Autodesk Inventor part; units mm, degrees
ref_plane "YZ Plane" through (0, 0, 0) normal (1, 0, 0) x (0, 1, 0)
ref_plane "XZ Plane" through (0, 0, 0) normal (0, 1, 0) x (-1, 0, 0)
ref_plane "XY Plane" through (0, 0, 0) normal (0, 0, 1) x (1, 0, 0)
sketch "Skizze4" plane through (0, 0, 0) normal (0, 1, 0) x (-1, 0, 0)
  line L0 (28.9949, 70) -> (70, 28.9949)
  line L1 (70, 28.9949) -> (70, -28.9949)
  line L2 (70, -28.9949) -> (28.9949, -70)
  line L3 (28.9949, -70) -> (-28.9949, -70)
  line L4 (-28.9949, -70) -> (-70, -28.9949)
  line L5 (-70, -28.9949) -> (-70, 28.9949)
  line L6 (-70, 28.9949) -> (-28.9949, 70)
  line L7 (-28.9949, 70) -> (28.9949, 70)
  line L8 (0, -98) -> (0, 98) construction
  line L9 (98, 0) -> (-98, 0) construction
  point P0 (0, 0)
  point P1 (0, 0)
  dimension "d4" = 140
extrude "Extrusion2" add sketch "Skizze4" along normal blind 2.5
sketch "Skizze9" plane through (0, 2.5, 0) normal (0, 1, 0) x (1, 0, 0)
  line L0 (-70, -28.9949) -> (-28.9949, -70) construction
  line L1 (-28.9949, -70) -> (28.9949, -70) construction
  line L2 (28.9949, -70) -> (70, -28.9949) construction
  line L3 (70, -28.9949) -> (70, 28.9949) construction
  line L4 (70, 28.9949) -> (28.9949, 70) construction
  line L5 (28.9949, 70) -> (-28.9949, 70) construction
  line L6 (-28.9949, 70) -> (-70, 28.9949) construction
  line L7 (-70, 28.9949) -> (-70, -28.9949) construction
  line L8 (-27.7523, -67) -> (-67, -27.7523)
  line L9 (-67, -27.7523) -> (-67, 27.7523)
  line L10 (-67, 27.7523) -> (-27.7523, 67)
  line L11 (-27.7523, 67) -> (27.7523, 67)
  line L12 (27.7523, 67) -> (67, 27.7523)
  line L13 (67, 27.7523) -> (67, -27.7523)
  line L14 (67, -27.7523) -> (27.7523, -67)
  line L15 (27.7523, -67) -> (-27.7523, -67)
  line L16 (-64, -26.5097) -> (-26.5097, -64)
  line L17 (-26.5097, -64) -> (26.5097, -64)
  line L18 (26.5097, -64) -> (64, -26.5097)
  line L19 (64, -26.5097) -> (64, 26.5097)
  line L20 (64, 26.5097) -> (26.5097, 64)
  line L21 (26.5097, 64) -> (-26.5097, 64)
  line L22 (-26.5097, 64) -> (-64, 26.5097)
  line L23 (-64, 26.5097) -> (-64, -26.5097)
  point P0 (0, 0)
  dimension "d20" = 3
  dimension "d21" = 3
extrude "Extrusion6" add sketch "Skizze9" along normal blind 3
sketch "Skizze7" plane through (0, 0, 0) normal (0, -1, 0) x (1, 0, 0)
  line L0 (-28.9949, 70) -> (-70, 28.9949) construction
  line L1 (-70, 28.9949) -> (-70, -28.9949) construction
  line L2 (-70, -28.9949) -> (-28.9949, -70) construction
  line L3 (-28.9949, -70) -> (28.9949, -70) construction
  line L4 (28.9949, -70) -> (70, -28.9949) construction
  line L5 (70, -28.9949) -> (70, 28.9949) construction
  line L6 (70, 28.9949) -> (28.9949, 70) construction
  line L7 (28.9949, 70) -> (-28.9949, 70) construction
  line L8 (-70, 28.9949) -> (-70, -28.9949)
  arc A0 (-70, 9.798) -> (-70, -9.798) centre (-60, 0) ccw
  line L9 (-87.767, 0) -> (-49.4975, 0) construction
  line L10 (-78.3477, 9.798) -> (-61.6523, 9.798) construction
  line L11 (-77.7764, -9.798) -> (-65.8218, -9.798) construction
  line L12 (-119.3204, 0) -> (101.5534, 0) construction
  point P0 (0, 0)
  dimension "d15" = 14
  dimension "d16" = 10
extrude "Extrusion5" add sketch "Skizze7" against normal up to surface (2.5 mm away)
properties part number "Oktagon_Deckel" material "Kst - PC/Makrolon (clear)"
Source: CAD feature listing. Evaluate the final solid. Frame: model axes, mm. A direction names the side the tool comes from. Give positions to 0.01 mm unless a question says otherwise; leave off trailing zeros. Write each loop counter-clockwise with the first axis right and the second up, starting at its lowest first coordinate (ties: lowest second). Pieces come first, ordered by that corner, then holes.
1. First-contact query: pin 1 (1.5 mm diameter, centred on y = 4.5, z = 10.5, fed in from -X); pin 2 (3 mm diameter, centred on x = -43.5, z = 31, fed in from +Y); pin 3 (10 mm diameter, centred on x = 22.5, z = -53.5, fed in from -Y); pin 4 (1.5 mm diameter, centred on x = 13, y = 3.5, fed in from +Z). Flat tips, straight axial feed; report the tip coordinate or a pass-through.
2. Section query C-C (x = 23.5). Return the cut outline in (y, z), then the cut area to 3 significant figures.
3. Section query B-B (z = 18.5). Return the cut outline in (x, y), then the cut area to 3 significant figures.
4. Pull-direction query (X, two-part tool) for faces 1 (the face through (44.99, 3.98, 45.52)), 2 (the face through (-47.65, 3.98, -47.1)), 3 (the face through (49, 5.5, 44)); classes: +X half, -X half, draft (parallel to the pull), parting line (faces both ways), or undercut.
5. Section query A-A (y = 4.35). Return the cut outline in (x, z).
6. Material intervals for line 1 along Z through (x, y) = (20, 4.6); line 2 along Y through (x, z) = (36, 10.5), sorted ascending.
7. Access query for faces 4 (the face through (47.65, 3.98, 47.1)), 5 (the face through (-44.99, 3.98, -45.52)), 6 (the face through (-47.1, 3.98, 47.65)). Directions: +Z, -Z, +X, -X, +Y, -Y. A direction counts if a zero-diameter tool reaches every point of the face in a straight line with its end or side. Return the directions, or none.
Output values:
1. pin 1: stops at x = -67
1. pin 2: stops at y = 2.5
1. pin 3: stops at y = 0
1. pin 4: stops at z = 67
2. outline: (0, -70) - (2.5, -70) - (2.5, -67) - (5.5, -67) - (5.5, -64) - (2.5, -64) - (2.5, 64) - (5.5, 64) - (5.5, 67) - (2.5, 67) - (2.5, 70) - (0, 70) - close
2. area: 368 mm2
3. outline: (-70, 0) - (70, 0) - (70, 2.5) - (67, 2.5) - (67, 5.5) - (64, 5.5) - (64, 2.5) - (-64, 2.5) - (-64, 5.5) - (-67, 5.5) - (-67, 2.5) - (-70, 2.5) - close
3. area: 368 mm2
4. face 1: undercut
4. face 2: -X half
4. face 3: draft
5. outline: (-67, -27.75) - (-27.75, -67) - (27.75, -67) - (67, -27.75) - (67, 27.75) - (27.75, 67) - (-27.75, 67) - (-67, 27.75) - close; hole (-64, -26.51) - (-26.51, -64) - (26.51, -64) - (64, -26.51) - (64, 26.51) - (26.51, 64) - (-26.51, 64) - (-64, 26.51) - close
6. line 1: z = -67 to -64, 64 to 67
6. line 2: y = 0 to 2.5
7. face 4: +Z, +X, +Y
7. face 5: +Y
7. face 6: +Z, -X, +Y
